```python
from build123d import *
from build123d.topology import SkipClean

# Parameters (mm, degrees)
SKETCH1_R           = 2.5
BOSS_EXTRUDE1_DEPTH = 5
SKETCH2_R           = 28
SKETCH2_R_2         = 26


with BuildPart() as part:
    # Sketch1 → Boss-Extrude1 (new body)
    with BuildSketch(Plane.XY):
        with BuildLine():
            Line((0, 30), (0, 26))
            ThreePointArc((0, 26), (-26, 0), (0, -26))
            Line((0, -26), (0, -30))
            ThreePointArc((0, -30), (-17.439949034, -24.410001591), (-28.380612245, -9.723211846))
            ThreePointArc((-28.380612245, -9.723211846), (-30.5492718, -7.049680039), (-33.932142857, -6.411683174))
            ThreePointArc((-33.932142857, -6.411683174), (-41.5, 0), (-33.932142857, 6.411683174))
            ThreePointArc((-33.932142857, 6.411683174), (-30.5492718, 7.049680039), (-28.380612245, 9.723211846))
            ThreePointArc((-28.380612245, 9.723211846), (-17.439949034, 24.410001591), (0, 30))
        make_face()
        with Locations((-35, 0)):
            Circle(SKETCH1_R, mode=Mode.SUBTRACT)
    boss_extrude1 = extrude(amount=BOSS_EXTRUDE1_DEPTH)

    # Mirror1: Boss-Extrude1 across plane
    add(boss_extrude1.mirror(Plane(origin=(0, 30, 5), x_dir=(0, 0, 1), z_dir=(-1, 0, 0))))

    # Sweep1: sweep along a path in Sketch3
    with SkipClean():  # the faces are left unmerged after this step: merging them gives an invalid solid
        with BuildLine(Plane(origin=(0, 0, 0), x_dir=(0, 0, -1), z_dir=(1, 0, 0))) as sweep1_path:
            Line((-5, 0), (-50, 0))
            ThreePointArc((-50, 0), (-85.355339059, -14.644660941), (-100, -50))
            Line((-100, -50), (-100, -200))
        # Sketch2 → Sweep1 (sweep)
        with BuildSketch(Plane.XY.offset(5)):
            Circle(SKETCH2_R)
            Circle(SKETCH2_R_2, mode=Mode.SUBTRACT)
        sweep(path=sweep1_path.line)


solid = part.part
```
CAD build for the part. Positions are in the model's coordinates, mm. A direction names the side the tool comes from. Coordinates: 2 decimals unless noted, no trailing zeros. Loops run counter-clockwise (first coordinate to the right, second up) from the corner with the lowest first, then second, coordinate; pieces in that order, holes last. Notation, with made-up numbers: (30.25, 28.5) - (65.25, 28.5) arc R22 cw to (65.25, 49.5) - close; hole circle Ø4 at (-36.75, -19). An arc over 180 degrees is marked (long way). Use CSV: the item, a comma, the result in double quotes. Start each with the question number.
Q1. Probe probe 1 along Y at (x, z) = (0, 33); probe 2 along Z at (x, y) = (0, -111.5); probe 3 along Y at (x, z) = (35, 2). List the from-to ranges inside material, lowest first. Write a range as from..to.
Q2. Cut at B-B, the plane y = 0. State how many separate pieces and enclosed holes the cut face has, then the cut area to 3 significant figures.
Q3. Cut at D-D, the plane y = -88.5. List the corners of the cut face in (x, z), then the cut area to 3 significant figures.
Q4. Cut at A-A, the plane x = 4.5. List the corners of the cut face in (y, z), then the cut area to 3 significant figures.
Q5. Drop flat-ended pins along their axis: P1, Ø6, axis at x = 35, y = 0, coming from the -Z side; P2, Ø5, axis at x = -28, y = -151.5, coming from the -Z side; P3, Ø5, axis at x = 14.5, y = -1, coming from the +Z side; P4, Ø8, axis at x = 24.5, y = -117, coming from the +Z side. Give the stop position or say it passes through.
Q6. 3-axis set-ups, long thin cutter, end or side, ignore diameter. For faces 1 (the cylindrical face through (25.865, -10.724, 27.815)), 2 (the cylindrical face through (-30.507, -7.075, 2.465)): which of +Z, -Z, +X, -X, +Y, -Y reach the whole face in a straight line?
Q7. Cut at C-C, the plane z = 37. List the corners of the cut face in (x, y), then the cut area to 3 significant figures.
Q8. Two-plate mould, pull along X, no slides. Class faces 3 (the cylindrical face through (-3.38, -126.05, 125.78)), 4 (the flat face through (-28, 5, 5)), 5 (the cylindrical face through (-6.07, -126.05, 72.666)): +X half, -X half, draft (parallel to the pull), parting line (faces both ways), or undercut.
Here are the results:
1,probe 1,"-28..-26, 26..28"
1,probe 2,"72..74, 126..128"
1,probe 3,"-6.5..-2.5, 2.5..6.5"
2,separate pieces,"3"
2,enclosed holes,"0"
2,area,"604 mm2"
3,outline,"circle Ø56 at (0, 100); hole circle Ø52 at (0, 100)"
3,area,"339 mm2"
4,outline,"(-200, 72.36) - (-50, 72.36) arc R22.36 cw to (-27.64, 50) - (-27.64, 5) - (-29.66, 5) - (-29.66, 0) - (-25.61, 0) - (-25.61, 50) arc R24.39 ccw to (-50, 74.39) - (-200, 74.39) - close; (-200, 125.61) - (-50, 125.61) arc R75.61 cw to (25.61, 50) - (25.61, 0) - (29.66, 0) - (29.66, 5) - (27.64, 5) - (27.64, 50) arc R77.64 ccw to (-50, 127.64) - (-200, 127.64) - close"
4,area,"1,150 mm2"
5,P1,"z = 0"
5,P2,"z = 88.43"
5,P3,"z = 108.19"
5,P4,"z = 119.07"
6,face 1,"none"
6,face 2,"+Z, -Z, -Y"
7,outline,"circle Ø56 at (0, 0); hole circle Ø52 at (0, 0)"
7,area,"339 mm2"
8,face 3,"undercut"
8,face 4,"draft"
8,face 5,"parting line"
